For this review, use the dimensioned drawing (mm, ordinates from the lowest corner) and the shaded views. A direction names the side the tool comes from. Coordinates: 2 decimals unless noted, no trailing zeros. Loops run counter-clockwise (first coordinate to the right, second up) from the corner with the lowest first, then second, coordinate; pieces in that order, holes last. Notation, with made-up numbers: M -4,8.5 L 43,8.5 A21 ccw 43,44.5 Z; hole C 14,-35 d4. An arc over 180 degrees is marked long. Write item = value, one per line.
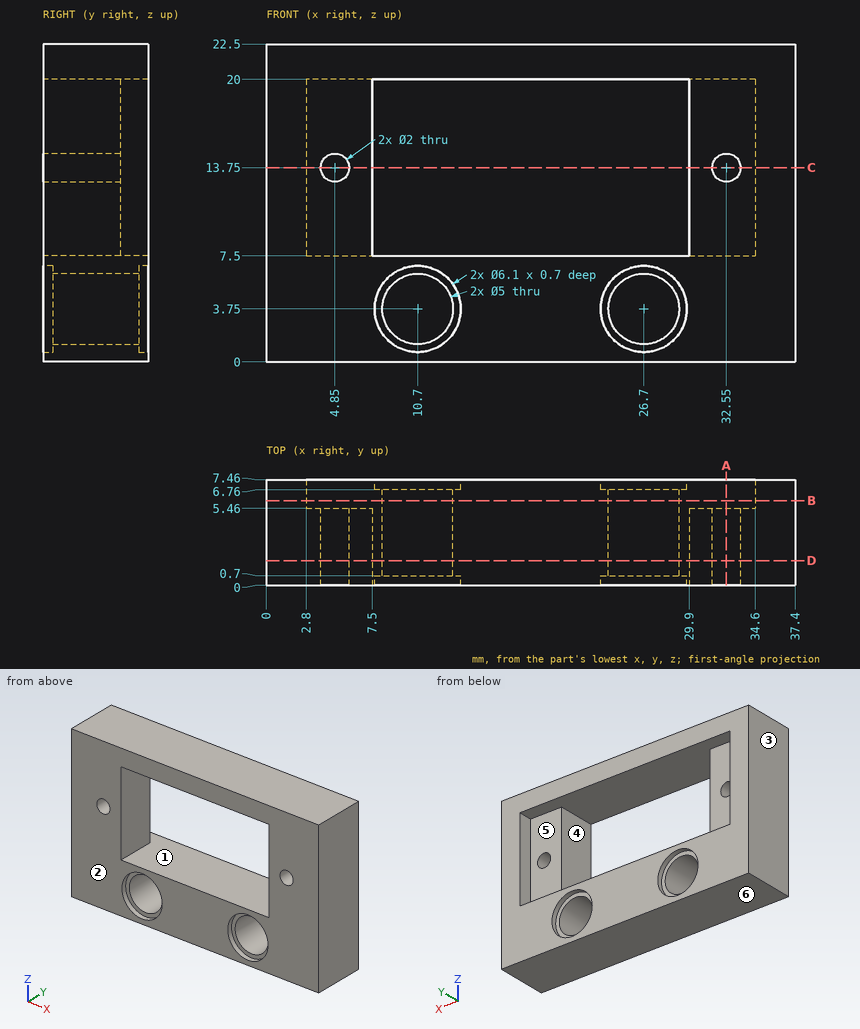
Q1. Add section A-A (x = 32.55). Write out the cut boundary in (y, z).
Solved:
outline = M 0,0 L 7.46,0 L 7.46,7.5 L 5.46,7.5 L 5.46,12.75 L 0,12.75 Z; M 0,14.75 L 5.46,14.75 L 5.46,20 L 7.46,20 L 7.46,22.5 L 0,22.5 Z
Q2. Add section B-B (y = 6). Write out the cut boundary in (x, z), and give its area (3 significant figures).
Solved:
outline = M 0,0 L 37.4,0 L 37.4,22.5 L 0,22.5 Z; hole M 2.8,7.5 L 34.6,7.5 L 34.6,20 L 2.8,20 Z; hole C 10.7,3.75 d5; hole C 26.7,3.75 d5
area = 405 mm²
Q3. For pin 1 Ø1.5 at (y, z) = (3.5, 17.5) entering from -X; pin 2 Ø3.5 at (x, z) = (10.7, 3.75) entering from -Y; pin 3 Ø2.5 at (x, z) = (32.55, 13.75) entering from +Y; pin 4 Ø6 at (x, z) = (10.7, 3.75) entering from -Y, all flat-tipped, find the tip position at first contact; note any pin that passes through.
Solved:
pin_1 = 0
pin_2 = through
pin_3 = 5.46
pin_4 = 0.7
Q4. Machinability: for the marked faces 4, 5 and 6, which of the approach directions +Z, -Z, +X, -X, +Y, -Y give a long, thin tool a straight path to every point of the face, cutting with its end or side? Answer none if there is none.
Solved:
face_4 = +Y, -Y
face_5 = +Y
face_6 = -Z, +X, -X, +Y, -Y
Q5. Draft analysis for pull direction X (two halves, no side actions). For the marked faces 1, 2 and 3, state which applies: +X half, -X half, draft (parallel to the pull), parting line (faces both ways), or undercut.
Solved:
face_1 = undercut
face_2 = draft
face_3 = -X half
Q6. Add section D-D (y = 1.75). Write out the cut boundary in (x, z).
Solved:
outline = M 0,0 L 37.4,0 L 37.4,22.5 L 0,22.5 Z; hole C 4.85,13.75 d2; hole M 7.5,7.5 L 29.9,7.5 L 29.9,20 L 7.5,20 Z; hole C 10.7,3.75 d5; hole C 26.7,3.75 d5; hole C 32.55,13.75 d2
Q7. Add section C-C (z = 13.75). Write out the cut boundary in (x, y), and give its area (3 significant figures).
Solved:
outline = M 0,0 L 3.85,0 L 3.85,5.46 L 2.8,5.46 L 2.8,7.46 L 0,7.46 Z; M 5.85,0 L 7.5,0 L 7.5,5.46 L 5.85,5.46 Z; M 29.9,0 L 31.55,0 L 31.55,5.46 L 29.9,5.46 Z; M 33.55,0 L 37.4,0 L 37.4,7.46 L 34.6,7.46 L 34.6,5.46 L 33.55,5.46 Z
area = 71.3 mm²
Q8. For line 1 along Z through (x, y) = (10.7, 0.45); line 2 along X through (y, z) = (4.25, 13.75); line 3 along Z through (x, y) = (8, 7.25), list the stretches that pass through material, from the lowest coordinate up.
Solved:
line_1 = 0 to 0.7, 6.8 to 7.5, 20 to 22.5
line_2 = 0 to 3.85, 5.85 to 7.5, 29.9 to 31.55, 33.55 to 37.4
line_3 = 0 to 2.33, 5.17 to 7.5, 20 to 22.5
